```python
from build123d import *

# Parameters (mm, degrees)
SKETCH1_W                   = 25.8064
SKETCH1_H                   = 25.8064
BOSS_EXTRUDE1_DEPTH         = 1.5875
SKETCH2_W                   = 13.1064
SKETCH2_H                   = 13.1064
BOSS_EXTRUDE2_DEPTH         = 1.27
F_32_0_116_DIAMETER_HOLE1_D = 2.9464


with BuildPart() as part:
    # Sketch1 → Boss-Extrude1 (new body)
    with BuildSketch(Plane(origin=(0, 0, 0), x_dir=(1, 0, 0), z_dir=(0, 1, 0))):
        Rectangle(SKETCH1_W, SKETCH1_H)
    extrude(amount=BOSS_EXTRUDE1_DEPTH)

    # Sketch2 → Boss-Extrude2 (add)
    with BuildSketch(Plane(origin=(0, 1.5875, 0), x_dir=(1, 0, 0), z_dir=(0, 1, 0))):
        Rectangle(SKETCH2_W, SKETCH2_H)
    extrude(amount=BOSS_EXTRUDE2_DEPTH)

    # #32 (0.116) Diameter Hole1 (through all)
    with Locations(Plane(origin=(-9.7282, 1.5875, -9.7282), x_dir=(0, 0, 1), z_dir=(0, 1, 0))):
        with Locations((0, 0), (19.4564, 0), (19.4564, 19.4564), (0, 19.4564)):
            Hole(F_32_0_116_DIAMETER_HOLE1_D / 2)


solid = part.part
```
Read the model definition and answer for the solid it produces. Units are mm, in the model's axes. A direction names the side the tool comes from. Round coordinates to 2 decimals unless told otherwise and drop trailing zeros. Write each loop counter-clockwise with the first axis right and the second up, starting at its lowest first coordinate (ties: lowest second). Pieces come first, ordered by that corner, then holes. Notation, with made-up numbers: (36, -7.5) -> (43, -7.5) arc R23 ccw to (43, 25.5) -> close; hole circle Ø4 at (18, 44). An arc over 180 degrees is marked (long way). Answer in a Markdown table with one row per item. Add a question column.
1) Find section B-B, the plane z = 3.5. Determine the outline of the cut face in (x, y).
2) Find section D-D, the plane z = -9.5. Determine the outline of the cut face in (x, y), and give its area (3 significant figures).
3) Which of the six approach directions +Z, -Z, +X, -X, +Y, -Y give full straight-line access (tool end or side, diameter ignored) to faces 1 (the face through (6.553, 2, 0)), 2 (the face through (0, 2, -6.553)), 3 (the face through (0, 2, 6.553)), 4 (the face through (12.903, 1, 0)), 5 (the face through (-9.663, 0.783, -8.256))?
4) Find section C-C, the plane y = 1. Determine the outline of the cut face in (x, z) (3 decimals).
5) Consider line 1 (X direction, y = 0.2, z = -9.75); line 2 (Y direction, x = -6.5, z = 7.25); line 3 (X direction, y = 2.4, z = 1.75). Determine where each line is inside the solid, lowest interval first.
6) Given P1, Ø1.8, axis at x = 9.73, z = -9.73, coming from the -Y side; P2, Ø3, axis at x = -4, z = 1, coming from the -Y side; P3, Ø1.4, axis at y = 2.5, z = 1.5, coming from the -X side; P4, Ø0.6, axis at y = 2, z = -1.5, coming from the +X side, each flat-ended and moving along its own axis, determine where each tip first touches the part or whether it passes through.
7) Determine the mould class of faces 6 (the face through (-8.486, 0.783, 8.936)), 7 (the face through (-6.553, 2, 0)), 8 (the face through (0, 0, 0)) for opening direction X: pulls with the +X half, pulls with the -X half, needs draft (parallel to the pull), parting line crosses it, or undercut.
8) Find section A-A, the plane x = 4.5. Determine the outline of the cut face in (y, z), and give its area (3 significant figures).
Findings below:
| question | item | result |
|---|---|---|
| 1 | outline | (-12.9, 0) -> (12.9, 0) -> (12.9, 1.59) -> (6.55, 1.59) -> (6.55, 2.86) -> (-6.55, 2.86) -> (-6.55, 1.59) -> (-12.9, 1.59) -> close |
| 2 | outline | (-12.9, 0) -> (-11.18, 0) -> (-11.18, 1.59) -> (-12.9, 1.59) -> close; (-8.27, 0) -> (8.27, 0) -> (8.27, 1.59) -> (-8.27, 1.59) -> close; (11.18, 0) -> (12.9, 0) -> (12.9, 1.59) -> (11.18, 1.59) -> close |
| 2 | area | 31.7 mm² |
| 3 | face 1 | +Z, -Z, +X, +Y |
| 3 | face 2 | -Z, +X, -X, +Y |
| 3 | face 3 | +Z, +X, -X, +Y |
| 3 | face 4 | +Z, -Z, +X, +Y, -Y |
| 3 | face 5 | +Y, -Y |
| 4 | outline | (-12.903, -12.903) -> (12.903, -12.903) -> (12.903, 12.903) -> (-12.903, 12.903) -> close; hole circle Ø2.946 at (-9.728, -9.728); hole circle Ø2.946 at (-9.728, 9.728); hole circle Ø2.946 at (9.728, -9.728); hole circle Ø2.946 at (9.728, 9.728) |
| 5 | line 1 | -12.9 to -11.2, -8.26 to 8.26, 11.2 to 12.9 |
| 5 | line 2 | 0 to 1.59 |
| 5 | line 3 | -6.55 to 6.55 |
| 6 | P1 | through |
| 6 | P2 | y = 0 |
| 6 | P3 | x = -6.55 |
| 6 | P4 | x = 6.55 |
| 7 | face 6 | undercut |
| 7 | face 7 | pulls with the -X half |
| 7 | face 8 | needs draft |
| 8 | outline | (0, -12.9) -> (1.59, -12.9) -> (1.59, -6.55) -> (2.86, -6.55) -> (2.86, 6.55) -> (1.59, 6.55) -> (1.59, 12.9) -> (0, 12.9) -> close |
| 8 | area | 57.6 mm² |
